Input: part model. Units: mm. Frame: model coordinates. Face numbers are marked on the shaded views. A direction names the side the tool comes from. Coordinates: 2 decimals unless noted, no trailing zeros. Order: outer loops, then holes, each group sorted by start corner. A loop starts at its lowest first (then second) coordinate and runs counter-clockwise, first axis right, second up. Notation, with made-up numbers: (41, -1.5) -> (81, -1.5) arc R34 ccw to (81, 34.5) -> close; hole circle Ø3 at (84.5, -17). An arc over 180 degrees is marked (long way). One line per question, with ' | ' between items.
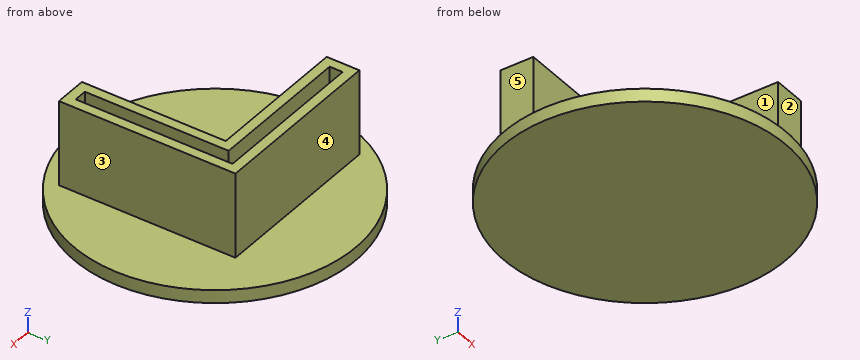
```python
from build123d import *

# Parameters (mm, degrees)
F0_R     = 21.5576072156
F1_DEPTH = 2
F2_DEPTH = 15


with BuildPart() as f1:
    # F0 (on Top) → F1 (new body)
    with BuildSketch(Plane.XY):
        with Locations((3, 3)):
            Circle(F0_R)
        Polygon((-13.5, 13.5), (13.5, 13.5), (13.5, -13.5), (8.5, -13.5), (8.5, -8.5), (8.5, 8.5), (-8.5, 8.5), (-13.5, 8.5), align=None, mode=Mode.SUBTRACT)
        Polygon((13.5, -13.5), (13.5, 13.5), (-13.5, 13.5), (-13.5, 8.5), (-8.5, 8.5), (8.5, 8.5), (8.5, -8.5), (8.5, -13.5), align=None)
        Polygon((-12, 10), (-12, 12), (12, 12), (12, -12), (10, -12), (10, -10), (10, 10), (-10, 10), align=None, mode=Mode.SUBTRACT)
        Polygon((12, 12), (-12, 12), (-12, 10), (-10, 10), (10, 10), (10, -10), (10, -12), (12, -12), align=None)
    extrude(amount=F1_DEPTH)

    # F0 (on Top) → F2 (join)
    with BuildSketch(Plane.XY):
        Polygon((13.5, -13.5), (13.5, 13.5), (-13.5, 13.5), (-13.5, 8.5), (-8.5, 8.5), (8.5, 8.5), (8.5, -8.5), (8.5, -13.5), align=None)
        Polygon((-12, 10), (-12, 12), (12, 12), (12, -12), (10, -12), (10, -10), (10, 10), (-10, 10), align=None, mode=Mode.SUBTRACT)
    extrude(amount=F2_DEPTH)


solid = f1.part
```
1. Cut plane D-D, the plane x = 20. Return loops of the section in (y, z), and give its area (3 significant figures).
Recorded:
outline: (-10.26, 0) -> (16.26, 0) -> (16.26, 2) -> (-10.26, 2) -> close | area: 53.0 mm^2
2. Cut plane B-B, the plane y = 3. Return loops of the section in (x, z).
Recorded:
outline: (-18.56, 0) -> (24.56, 0) -> (24.56, 2) -> (13.5, 2) -> (13.5, 15) -> (12, 15) -> (12, 2) -> (10, 2) -> (10, 15) -> (8.5, 15) -> (8.5, 2) -> (-18.56, 2) -> close
3. Cut plane A-A, the plane z = 5. Return loops of the section in (x, y).
Recorded:
outline: (-13.5, 8.5) -> (8.5, 8.5) -> (8.5, -13.5) -> (13.5, -13.5) -> (13.5, 13.5) -> (-13.5, 13.5) -> close; hole (-12, 10) -> (10, 10) -> (10, -12) -> (12, -12) -> (12, 12) -> (-12, 12) -> close
4. Pin query (flat end, axial travel): pin 1 Ø12 at (x, y) = (13.5, 10.5) entering from -Z; pin 2 Ø2 at (x, z) = (-11, 10.5) entering from -Y; pin 3 Ø1.5 at (y, z) = (10.5, 9.5) entering from -X; pin 4 Ø1 at (y, z) = (10.5, 10) entering from +X. Return the tip coordinate at first contact, or that it passes through.
Recorded:
pin 1: stops at z = 0 | pin 2: stops at y = 8.5 | pin 3: stops at x = -13.5 | pin 4: stops at x = 13.5
5. Access query for the marked faces 1, 2, 3, 4 and 5. Directions: +Z, -Z, +X, -X, +Y, -Y. A direction counts if a zero-diameter tool reaches every point of the face in a straight line with its end or side. Return the directions, or none.
Recorded:
face 1: +Z, -X, -Y | face 2: +Z, +X, -X, -Y | face 3: +Z, +X, +Y, -Y | face 4: +Z, +X, -X, +Y | face 5: +Z, -X, +Y, -Y
6. Ray query, line 1 (X direction, y = -9.5, z = 14); line 2 (Z direction, x = 8, y = -4.5). Return the intervals inside material, ascending. Write a range as [from, to].
Recorded:
line 1: x = [8.5, 10], [12, 13.5] | line 2: z = [0, 2]
